Autodesk Inventor part; units mm, degrees
ref_plane "YZ Plane" through (0, 0, 0) normal (1, 0, 0) x (0, 1, 0)
ref_plane "XZ Plane" through (0, 0, 0) normal (0, 1, 0) x (-1, 0, 0)
ref_plane "XY Plane" through (0, 0, 0) normal (0, 0, 1) x (1, 0, 0)
sketch "スケッチ1" plane through (0, 0, 0) normal (1, 0, 0) x (0, 1, 0)
  line L0 (0, 0) -> (30, 0)
  line L1 (30, 0) -> (30, -30)
  line L2 (30, -30) -> (0, -30)
  line L3 (0, -30) -> (0, 0)
  circle A0 centre (25.253, -4.747) radius 1.25
  line L4 (15, 0) -> (15, -30)
  line L5 (30, -15) -> (0, -15)
  circle A1 centre (4.747, -4.747) radius 1.25
  circle A2 centre (25.253, -25.253) radius 1.25
  circle A3 centre (4.747, -25.253) radius 1.25
  line L6 (-2, 5) -> (3, 5)
  line L7 (3, 5) -> (3, -35)
  line L8 (3, -35) -> (-2, -35)
  line L9 (-2, -35) -> (-2, 5)
  line L10 (30, 0) -> (3, 5)
  line L11 (30, -30) -> (3, -35)
  circle A4 centre (15, -15) radius 10
  dimension "d0" = 30
  dimension "d1" = 30
  dimension "d2" = 2.5
  dimension "d3" = 4.747
  dimension "d4" = 4.747
  dimension "d5" = 5
  dimension "d6" = 2
  dimension "d7" = 5
  dimension "d8" = 5
  dimension "d12" = 20
extrude "押し出し1" add sketch "スケッチ1" against normal blind 5 contours L0 L7 L10 | L4 A4 L5 L7 L0 | L0 L1 L5 A4 L4 | L7 L5 L3 L0 | L0 L3 L2 L7 L8 L9 L6 | L1 L2 L4 A4 L5 | L7 L2 L3 L5 | L5 A4 L4 L2 L7 | L11 L7 L2
fillet "フィレット1" radius 2 4 edges at (-2.5, 30, 0) (-2.5, 3, 5) (-2.5, 30, -30) (-2.5, 3, -35)
sketch "スケッチ2" plane through (0, -2, -35) normal (0, -1, 0) x (1, 0, 0)
  line L0 (0, 0) -> (-5, 0)
  line L1 (-2.5, 0) -> (-2.5, 40)
  line L2 (0, 40) -> (-5, 40)
  point P0 (0, 35)
  point P1 (-2.5, 15)
  point P2 (-2.5, 25)
  dimension "d13" = 15
  dimension "d14" = 10
hole "穴1" at (-2.5, -2, -20) at (-2.5, -2, -10) direction (0, 1, 0) diameter 2.5 depth 5 tip angle 118
equation "\"d4\" = d3"
properties part number "belt_liner_v5_Plate_12" material "アルミニウム 6061"
Model file for the job. Use its own axes, mm. A direction names the side the tool comes from. Give positions to 0.01 mm unless a question says otherwise; leave off trailing zeros. Loops run counter-clockwise (first coordinate to the right, second up) from the corner with the lowest first, then second, coordinate; pieces in that order, holes last.
1) Saw through at C-C (z = 2.5). Write the cut outline in (x, y).
2) Saw through at D-D (x = -3). Count the separate pieces of the cut face and the enclosed holes in it, plus the area to 3 significant figures.
3) Saw through at A-A (z = -15). Write the cut outline in (x, y), plus the area to 3 significant figures.
4) Wall check: line 1 (X direction, y = 0.8, z = -10); line 2 (Z direction, x = -1.45, y = -1); line 3 (Y direction, x = -1.45, z = -4.5). Give the ranges that are in metal, low to high.
5) Flat gauge pin, fed straight in: pin 1 Ø2 at (x, y) = (-3, 13) entering from -Z. Where does the tip first touch, or does it go through?
6) Saw through at B-B (y = 0). Write the cut outline in (x, z), plus the area to 3 significant figures.
7) Pull direction Y, two halves, no side cores. Call faces 3 (the cylindrical face through (-2.46, 4.58, -3.51)), 4 (the cylindrical face through (-2.46, 24.54, -12)), 5 (the flat face through (-2, -2, -15)), 6 (the flat face through (-2, 30, -15)): +Y half, -Y half, draft (parallel to the pull), parting line (faces both ways), or undercut.
8) Tool access for faces 1 (the flat face through (0, 3, -15)), 2 (the cylindrical face through (-2.021, 0.535, -21.155)): list every direction of +Z, -Z, +X, -X, +Y, -Y with a clear straight run to the whole face (end or side of a thin tool).
Answer block:
1. outline: (-5, -2) - (0, -2) - (0, 16.5) - (-5, 16.5) - close
2. separate pieces: 1
2. enclosed holes: 5
2. area: 786 mm2
3. outline: (-5, -2) - (0, -2) - (0, 5) - (-5, 5) - close; (-5, 25) - (0, 25) - (0, 30) - (-5, 30) - close
3. area: 60.0 mm2
4. line 1: x = -5 to -3.75, -1.25 to 0
4. line 2: z = -35 to -20.68, -19.32 to -10.68, -9.32 to 5
4. line 3: y = -2 to 3.52, 5.97 to 24.03, 26.48 to 30
5. pin 1: stops at z = -33.33
6. outline: (-5, -35) - (0, -35) - (0, 5) - (-5, 5) - close; hole circle Ø2.5 at (-2.5, -20); hole circle Ø2.5 at (-2.5, -10)
6. area: 190 mm2
7. face 3: undercut
7. face 4: undercut
7. face 5: -Y half
7. face 6: +Y half
8. face 1: +Z, -Z, +X, +Y, -Y
8. face 2: -Y
